```python
from build123d import *

# Parameters (mm, degrees)
ESBO_O1_R                = 1.5
RESSALTO_EXTRUS_O1_DEPTH = 1.5


with BuildPart() as part:
    # Esboço1 → Ressalto-extrusão1 (new body)
    with BuildSketch(Plane(origin=(0, 0, 0), x_dir=(1, 0, 0), z_dir=(0, 1, 0))):
        with BuildLine():
            Line((-5, -3.75), (-5, 1.75))
            ThreePointArc((-5, 1.75), (-4.414213562, 3.164213562), (-3, 3.75))
            Line((-3, 3.75), (3, 3.75))
            ThreePointArc((3, 3.75), (4.414213562, 3.164213562), (5, 1.75))
            Line((5, 1.75), (5, -3.75))
            Line((5, -3.75), (-5, -3.75))
        make_face()
        with Locations(Location((0, 0.75, 0), (0, 0, 270))):
            Circle(ESBO_O1_R, mode=Mode.SUBTRACT)
    extrude(amount=RESSALTO_EXTRUS_O1_DEPTH)


solid = part.part
```
The model under review builds one solid part; all positions refer to its coordinate system, in mm. Coordinates: 2 decimals unless noted, no trailing zeros. Order: outer loops, then holes, each group sorted by start corner. A loop starts at its lowest first (then second) coordinate and runs counter-clockwise, first axis right, second up. Notation, with made-up numbers: (-12, 36) -> (6, 36) arc R26 ccw to (6, 60) -> close; hole circle Ø7 at (51.25, 41.25). An arc over 180 degrees is marked (long way). Answer in a Markdown table with one row per item. Add a question column.
Item 1: To check wall thickness, follow probe 1 along X at (y, z) = (0.7, -0.75); probe 2 along Z at (x, y) = (0.5, 0.75); probe 3 along X at (y, z) = (0.55, 0.5). State the ranges of each line that lie inside material, in increasing order.
Item 2: We need section B-B on x = 1. Write out the cut boundary in (y, z), plus the area to 3 significant figures.
Item 3: We need section A-A on z = -0.75. Write out the cut boundary in (x, y).
Item 4: Mouldability with a two-part tool opening along X and no side actions: class faces 1 (the cylindrical face through (-0.91, 0.74, -1.94)), 2 (the flat face through (-5, 1, 1)), 3 (the flat face through (0, 0, 1)) as +X half, -X half, draft (parallel to the pull), parting line (faces both ways), or undercut.
Item 5: We need section C-C on y = 0.35. Write out the cut boundary in (x, z).
Final values:
| question | item | result |
|---|---|---|
| 1 | probe 1 | x = -5 to -1.5, 1.5 to 5 |
| 1 | probe 2 | z = -3.75 to -2.16, 0.66 to 3.75 |
| 1 | probe 3 | x = -5 to -0.83, 0.83 to 5 |
| 2 | outline | (0, -3.75) -> (1.5, -3.75) -> (1.5, -1.87) -> (0, -1.87) -> close; (0, 0.37) -> (1.5, 0.37) -> (1.5, 3.75) -> (0, 3.75) -> close |
| 2 | area | 7.90 mm2 |
| 3 | outline | (-5, 0) -> (-1.5, 0) -> (-1.5, 1.5) -> (-5, 1.5) -> close; (1.5, 0) -> (5, 0) -> (5, 1.5) -> (1.5, 1.5) -> close |
| 4 | face 1 | undercut |
| 4 | face 2 | -X half |
| 4 | face 3 | draft |
| 5 | outline | (-5, -1.75) arc R2 ccw to (-3, -3.75) -> (3, -3.75) arc R2 ccw to (5, -1.75) -> (5, 3.75) -> (-5, 3.75) -> close; hole circle Ø3 at (0, -0.75) |
